Could you check a few things on this model? Use its own coordinates, in mm. A direction names the side the tool comes from. Coordinates: 2 decimals unless noted, no trailing zeros. Write each loop counter-clockwise with the first axis right and the second up, starting at its lowest first coordinate (ties: lowest second). Pieces come first, ordered by that corner, then holes. Notation, with made-up numbers: M 70.5,38 L 96.5,38 A30 ccw 96.5,60 Z; hole C 82.5,-31 d9. An arc over 180 degrees is marked long. Write item = value, one per line.
```python
from build123d import *

# Parameters (mm, degrees)
SKETCH1_W           = 43.25
SKETCH1_H           = 5.00807777
BOSS_EXTRUDE1_DEPTH = 18
SKETCH2_W           = 33.5
SKETCH2_H           = 12
CUT_EXTRUDE1_DEPTH  = 4
CUT_EXTRUDE2_REACH  = 30.419
SKETCH3_W           = 25.5
SKETCH3_H           = 12
CUT_EXTRUDE3_REACH  = 30.419
SKETCH4_W           = 5
SKETCH4_H           = 5
BOSS_EXTRUDE2_DEPTH = 5.00807777


with BuildPart() as part:
    # Sketch1 → Boss-Extrude1 (new body)
    with BuildSketch(Plane.XY):
        with Locations((0, -2.504038885)):
            Rectangle(SKETCH1_W, SKETCH1_H)
    extrude(amount=BOSS_EXTRUDE1_DEPTH)

    # Sketch2 → Cut-Extrude1 (cut)
    with BuildSketch(Plane(origin=(0, 0, 0), x_dir=(1, 0, 0), z_dir=(0, 1, 0))):
        with Locations((0.875, -9)):
            Rectangle(SKETCH2_W, SKETCH2_H)
    extrude(amount=-CUT_EXTRUDE1_DEPTH, mode=Mode.SUBTRACT)

    # Sketch3 → Cut-Extrude2 (cut, up to next)
    with BuildSketch(Plane(origin=(0, -4, 0), x_dir=(1, 0, 0), z_dir=(0, 1, 0)), mode=Mode.PRIVATE) as cut_extrude2_sk1:
        with Locations((0.875, -9)):
            Rectangle(SKETCH3_W, SKETCH3_H)
    cut_extrude2_tool1 = extrude(cut_extrude2_sk1.sketch, amount=-CUT_EXTRUDE2_REACH, mode=Mode.PRIVATE) & part.part
    add(cut_extrude2_tool1.solids().sort_by_distance((0.875, -4, 9))[0], mode=Mode.SUBTRACT)

    # Sketch4 → Cut-Extrude3 (cut, up to next)
    with BuildSketch(Plane(origin=(0, -4, 0), x_dir=(1, 0, 0), z_dir=(0, 1, 0)), mode=Mode.PRIVATE) as cut_extrude3_sk1:
        with Locations((16.125, -9)):
            Rectangle(SKETCH4_W, SKETCH4_H)
    cut_extrude3_tool1 = extrude(cut_extrude3_sk1.sketch, amount=-CUT_EXTRUDE3_REACH, mode=Mode.PRIVATE) & part.part
    add(cut_extrude3_tool1.solids().sort_by_distance((16.125, -4, 9))[0], mode=Mode.SUBTRACT)

    # Sketch5 → Boss-Extrude2 (add)
    with BuildSketch(Plane(origin=(0, 0, 0), x_dir=(1, 0, 0), z_dir=(0, 1, 0))):
        Polygon((-21.625, 0), (-21.625, 3.721580372), (-17.903419628, 0), align=None)
        Polygon((-17.903419628, -18), (-21.625, -18), (-21.625, -21.721580372), align=None)
    extrude(amount=-BOSS_EXTRUDE2_DEPTH)


solid = part.part
```
Item 1: Imagine slicing it at C-C (x = -8.5). Write out the boundary of the cut face in (y, z), and give its area (3 significant figures).
Numbers:
outline = M -5.01,0 L 0,0 L 0,3 L -5.01,3 Z; M -5.01,15 L 0,15 L 0,18 L -5.01,18 Z
area = 30.0 mm²
Item 2: Imagine slicing it at A-A (y = -1.25). Write out the boundary of the cut face in (x, z) (3 decimals).
Numbers:
outline = M -21.625,-3.722 L -17.903,0 L 21.625,0 L 21.625,18 L -17.903,18 L -21.625,21.722 Z; hole M -15.875,3 L 17.625,3 L 17.625,15 L -15.875,15 Z
Item 3: Imagine slicing it at D-D (z = 4.75). Write out the boundary of the cut face in (x, y) (3 decimals), and give its area (3 significant figures).
Numbers:
outline = M -21.625,-5.008 L -11.875,-5.008 L -11.875,-4 L -15.875,-4 L -15.875,0 L -21.625,0 Z; M 13.625,-5.008 L 21.625,-5.008 L 21.625,0 L 17.625,0 L 17.625,-4 L 13.625,-4 Z
area = 56.9 mm²
Item 4: If we mould it in two halves opening along X, with no side actions, what happens to faces 1 (the face through (16.1, -4.5, 6.5)), 2 (the face through (-2, 0, 16)), 3 (the face through (-21.625, -2, 9)), 4 (the face through (1, -2, 15))? For each: pulls with the +X half, pulls with the -X half, needs draft (parallel to the pull), parting line crosses it, or undercut.
Numbers:
face_1 = undercut
face_2 = needs draft
face_3 = pulls with the -X half
face_4 = undercut
Item 5: For faces 5 (the face through (18, -4, 9)), 6 (the face through (13.625, -4.5, 4.8)), 7 (the face through (1, -2, 3)), which set-ups out of +Z, -Z, +X, -X, +Y, -Y let a thin tool reach every point of the face, with its end or its side?
Numbers:
face_5 = -Y
face_6 = +Y, -Y
face_7 = +Y
Item 6: I'm going to push flat-ended pins straight in: P1, Ø3, axis at x = 13, z = 9.5, coming from the -Y side; P2, Ø2.5, axis at x = 2, y = -3, coming from the +Z side; P3, Ø1.5, axis at x = 2.5, y = -2, coming from the -Z side; P4, Ø3, axis at x = -13, z = 11.5, coming from the +Y side. Where does each tip first touch, or does it pass through?
Numbers:
P1 = through
P2 = 18
P3 = 0
P4 = -4
Item 7: If I drill on line 1 along X through (y, z) = (-3.15, 5.5) (3 decimals); line 2 along Z through (x, y) = (-7, -1.2); line 3 along X through (y, z) = (-4.35, 14.75) (3 decimals), over which ranges is the centre line in solid material (lowest first)?
Numbers:
line_1 = -21.625 to -15.875, 17.625 to 21.625
line_2 = 0 to 3, 15 to 18
line_3 = -21.625 to -11.875, 13.625 to 21.625
Item 8: Imagine slicing it at B-B (z = 7.5). Write out the boundary of the cut face in (x, y) (3 decimals).
Numbers:
outline = M -21.625,-5.008 L -11.875,-5.008 L -11.875,-4 L -15.875,-4 L -15.875,0 L -21.625,0 Z; M 17.625,-4 L 18.625,-4 L 18.625,-5.008 L 21.625,-5.008 L 21.625,0 L 17.625,0 Z
